The model under review builds one solid part; all positions refer to its coordinate system, in mm. Round coordinates to 2 decimals unless told otherwise and drop trailing zeros. Order: outer loops, then holes, each group sorted by start corner. A loop starts at its lowest first (then second) coordinate and runs counter-clockwise, first axis right, second up. Notation, with made-up numbers: M -0.5,-3 L 11.5,-3 A16 cw 11.5,16 Z; hole C -3,44.5 d3. An arc over 180 degrees is marked long. Answer as a JSON object with one key per item and string values. Group by question number.
1) Consider section C-C, the plane z = -3.5. Write out the cut boundary in (x, y), then the cut area to 3 significant figures.
2) Consider section A-A, the plane y = 1.75. Count the separate pieces of the cut face and the enclosed holes in it, then the cut area to 3 significant figures.
3) Consider section B-B, the plane y = -0.25. Write out the cut boundary in (x, z).
4) To check wall thickness, follow line 1 (Y direction, x = 0.5, z = -1.5); line 2 (Z direction, x = 0, y = 6.5); line 3 (Z direction, x = -1.75, y = 3). State the ranges of each line that lie inside material, in increasing order.
5) Insertion check: pin 1 Ø3 at (x, y) = (0, 7) entering from -Z. The pin has a flat end and moves straight along its axis. Give the tip position at first contact, or say it passes through.
```python
from build123d import *

# Parameters (mm, degrees)
SKETCH3_R               = 0.25
SKETCH1_R               = 4
BOSS_EXTRUDE1_DEPTH     = 2
FILL_PATTERN2_OUTLINE_R = 0.25
FILL_PATTERN2_DEPTH     = 10


# Read off the part's stored shape, not the designer's step: Fill Pattern2
with BuildPart() as part:
    # Sweep1: sweep along a path in Sketch2
    with BuildLine(Plane(origin=(0, 0, 0), x_dir=(0, 0, -1), z_dir=(1, 0, 0))) as sweep1_path:
        Line((0, 0), (0, 10))
    # Sketch3 → Sweep1 (sweep)
    with BuildSketch(Plane(origin=(0, 0, 0), x_dir=(1, 0, 0), z_dir=(0, 1, 0))):
        Circle(SKETCH3_R)
    sweep(path=sweep1_path.line)

    # Sketch1 → Boss-Extrude1 (add)
    with BuildSketch(Plane(origin=(0, 0, 0), x_dir=(1, 0, 0), z_dir=(0, 1, 0))):
        with Locations(Location((0, 0, 0), (0, 0, 270))):
            Circle(SKETCH1_R)
    extrude(amount=-BOSS_EXTRUDE1_DEPTH)

    # Fill Pattern2 outline → Fill Pattern2 (add)
    with BuildSketch(Plane(origin=(0, 0, 0), x_dir=(1, 0, 0), z_dir=(0, 1, 0))):
        with Locations((-3.472963553, 0)):
            Circle(FILL_PATTERN2_OUTLINE_R)
        with Locations((-3.299315376, -0.984807753)):
            Circle(FILL_PATTERN2_OUTLINE_R)
        with Locations((-3.125667198, -1.969615506)):
            Circle(FILL_PATTERN2_OUTLINE_R)
        with Locations((-3.125667198, 1.969615506)):
            Circle(FILL_PATTERN2_OUTLINE_R)
        with Locations((-2.95201902, 0.984807753)):
            Circle(FILL_PATTERN2_OUTLINE_R)
        with Locations((-2.778370843, 0)):
            Circle(FILL_PATTERN2_OUTLINE_R)
        with Locations((-2.604722665, -0.984807753)):
            Circle(FILL_PATTERN2_OUTLINE_R)
        with Locations((-2.431074487, -1.969615506)):
            Circle(FILL_PATTERN2_OUTLINE_R)
        with Locations((-2.25742631, -2.954423259)):
            Circle(FILL_PATTERN2_OUTLINE_R)
        with Locations((-2.431074487, 1.969615506)):
            Circle(FILL_PATTERN2_OUTLINE_R)
        with Locations((-2.25742631, 0.984807753)):
            Circle(FILL_PATTERN2_OUTLINE_R)
        with Locations((-2.083778132, 0)):
            Circle(FILL_PATTERN2_OUTLINE_R)
        with Locations((-1.910129954, -0.984807753)):
            Circle(FILL_PATTERN2_OUTLINE_R)
        with Locations((-1.736481777, -1.969615506)):
            Circle(FILL_PATTERN2_OUTLINE_R)
        with Locations((-1.562833599, -2.954423259)):
            Circle(FILL_PATTERN2_OUTLINE_R)
        with Locations((-1.910129954, 2.954423259)):
            Circle(FILL_PATTERN2_OUTLINE_R)
        with Locations((-1.736481777, 1.969615506)):
            Circle(FILL_PATTERN2_OUTLINE_R)
        with Locations((-1.562833599, 0.984807753)):
            Circle(FILL_PATTERN2_OUTLINE_R)
        with Locations((-1.389185421, 0)):
            Circle(FILL_PATTERN2_OUTLINE_R)
        with Locations((-1.215537244, -0.984807753)):
            Circle(FILL_PATTERN2_OUTLINE_R)
        with Locations((-1.041889066, -1.969615506)):
            Circle(FILL_PATTERN2_OUTLINE_R)
        with Locations((-0.868240888, -2.954423259)):
            Circle(FILL_PATTERN2_OUTLINE_R)
        with Locations((-1.215537244, 2.954423259)):
            Circle(FILL_PATTERN2_OUTLINE_R)
        with Locations((-1.041889066, 1.969615506)):
            Circle(FILL_PATTERN2_OUTLINE_R)
        with Locations((-0.868240888, 0.984807753)):
            Circle(FILL_PATTERN2_OUTLINE_R)
        with Locations((-0.694592711, 0)):
            Circle(FILL_PATTERN2_OUTLINE_R)
        with Locations((-0.520944533, -0.984807753)):
            Circle(FILL_PATTERN2_OUTLINE_R)
        with Locations((-0.347296355, -1.969615506)):
            Circle(FILL_PATTERN2_OUTLINE_R)
        with Locations((-0.173648178, -2.954423259)):
            Circle(FILL_PATTERN2_OUTLINE_R)
        with Locations((-0.520944533, 2.954423259)):
            Circle(FILL_PATTERN2_OUTLINE_R)
        with Locations((-0.347296355, 1.969615506)):
            Circle(FILL_PATTERN2_OUTLINE_R)
        with Locations((-0.173648178, 0.984807753)):
            Circle(FILL_PATTERN2_OUTLINE_R)
        with Locations((0.173648178, -0.984807753)):
            Circle(FILL_PATTERN2_OUTLINE_R)
        with Locations((0.347296355, -1.969615506)):
            Circle(FILL_PATTERN2_OUTLINE_R)
        with Locations((0.520944533, -2.954423259)):
            Circle(FILL_PATTERN2_OUTLINE_R)
        with Locations((0.173648178, 2.954423259)):
            Circle(FILL_PATTERN2_OUTLINE_R)
        with Locations((0.347296355, 1.969615506)):
            Circle(FILL_PATTERN2_OUTLINE_R)
        with Locations((0.520944533, 0.984807753)):
            Circle(FILL_PATTERN2_OUTLINE_R)
        with Locations((0.694592711, 0)):
            Circle(FILL_PATTERN2_OUTLINE_R)
        with Locations((0.868240888, -0.984807753)):
            Circle(FILL_PATTERN2_OUTLINE_R)
        with Locations((1.041889066, -1.969615506)):
            Circle(FILL_PATTERN2_OUTLINE_R)
        with Locations((1.215537244, -2.954423259)):
            Circle(FILL_PATTERN2_OUTLINE_R)
        with Locations((0.868240888, 2.954423259)):
            Circle(FILL_PATTERN2_OUTLINE_R)
        with Locations((1.041889066, 1.969615506)):
            Circle(FILL_PATTERN2_OUTLINE_R)
        with Locations((1.215537244, 0.984807753)):
            Circle(FILL_PATTERN2_OUTLINE_R)
        with Locations((1.389185421, 0)):
            Circle(FILL_PATTERN2_OUTLINE_R)
        with Locations((1.562833599, -0.984807753)):
            Circle(FILL_PATTERN2_OUTLINE_R)
        with Locations((1.736481777, -1.969615506)):
            Circle(FILL_PATTERN2_OUTLINE_R)
        with Locations((1.910129954, -2.954423259)):
            Circle(FILL_PATTERN2_OUTLINE_R)
        with Locations((1.562833599, 2.954423259)):
            Circle(FILL_PATTERN2_OUTLINE_R)
        with Locations((1.736481777, 1.969615506)):
            Circle(FILL_PATTERN2_OUTLINE_R)
        with Locations((1.910129954, 0.984807753)):
            Circle(FILL_PATTERN2_OUTLINE_R)
        with Locations((2.083778132, 0)):
            Circle(FILL_PATTERN2_OUTLINE_R)
        with Locations((2.25742631, -0.984807753)):
            Circle(FILL_PATTERN2_OUTLINE_R)
        with Locations((2.431074487, -1.969615506)):
            Circle(FILL_PATTERN2_OUTLINE_R)
        with Locations((2.25742631, 2.954423259)):
            Circle(FILL_PATTERN2_OUTLINE_R)
        with Locations((2.431074487, 1.969615506)):
            Circle(FILL_PATTERN2_OUTLINE_R)
        with Locations((2.604722665, 0.984807753)):
            Circle(FILL_PATTERN2_OUTLINE_R)
        with Locations((2.778370843, 0)):
            Circle(FILL_PATTERN2_OUTLINE_R)
        with Locations((2.95201902, -0.984807753)):
            Circle(FILL_PATTERN2_OUTLINE_R)
        with Locations((3.125667198, -1.969615506)):
            Circle(FILL_PATTERN2_OUTLINE_R)
        with Locations((3.125667198, 1.969615506)):
            Circle(FILL_PATTERN2_OUTLINE_R)
        with Locations((3.299315376, 0.984807753)):
            Circle(FILL_PATTERN2_OUTLINE_R)
        with Locations((3.472963553, 0)):
            Circle(FILL_PATTERN2_OUTLINE_R)
    extrude(amount=FILL_PATTERN2_DEPTH)


solid = part.part
```
Results list:
{
 "1": {"outline": "M -1.94,-2 L 1.94,-2 L 1.94,0 L -1.94,0 Z", "area": "7.75 mm^2"},
 "2": {"separate pieces": "65", "enclosed holes": "0", "area": "12.8 mm^2"},
 "3": {"outline": "C 0,0 d8"},
 "4": {"line 1": "-2 to 0", "line 2": "-3.13 to -2.77, -1.16 to -0.8, -0.25 to 0.25, 0.8 to 1.16, 2.77 to 3.13", "line 3": "-3.15 to -2.76, -2.22 to -1.72, -1.15 to -0.82, 0.79 to 1.18, 1.72 to 2.22, 2.79 to 3.12"},
 "5": {"pin 1": "z = -3.2"}
}
